from build123d import *

# Parameters (mm, degrees)
SKETCH1_W            = 93
SKETCH1_H            = 100
BOSS_EXTRUDE2_DEPTH  = 10
SKETCH4_W            = 10.01
SKETCH4_H            = 15
BOSS_EXTRUDE4_DEPTH  = 24
SKETCH5_R            = 2
CUT_EXTRUDE1_DEPTH   = 50
SKETCH7_R            = 11
CUT_EXTRUDE3_DEPTH   = 50
SKETCH14_W           = 61.5
SKETCH14_H           = 42
CUT_EXTRUDE8_DEPTH   = 4
SKETCH19_R           = 11
CUT_EXTRUDE11_DEPTH  = 15
SKETCH20_R           = 2
CUT_EXTRUDE12_DEPTH  = 10
SKETCH21_W           = 40
SKETCH21_H           = 6
BOSS_EXTRUDE5_DEPTH  = 27
SKETCH22_W           = 40
SKETCH22_H           = 6.3
BOSS_EXTRUDE7_DEPTH  = 40
SKETCH23_R           = 8
CUT_EXTRUDE13_DEPTH  = 40
SKETCH24_W           = 118.277817783
SKETCH24_H           = 41.8
CUT_EXTRUDE14_DEPTH  = 40
SKETCH25_W           = 31.5
SKETCH25_H           = 23.2
CUT_EXTRUDE15_DEPTH  = 20
CUT_EXTRUDE18_DEPTH  = 3
SKETCH27_R           = 4.1
SKETCH27_R_2         = 4
CUT_EXTRUDE29_DEPTH  = 3
SKETCH28_W           = 29.5
SKETCH28_H           = 58.2
CUT_EXTRUDE30_DEPTH  = 23
SKETCH29_W           = 32
SKETCH29_H           = 4
CUT_EXTRUDE31_DEPTH  = 23
SKETCH31_W           = 32
SKETCH31_H           = 6
BOSS_EXTRUDE9_DEPTH  = 6.6
SKETCH32_W           = 32
SKETCH32_H           = 6
BOSS_EXTRUDE10_DEPTH = 10
SKETCH33_R           = 2
CUT_EXTRUDE32_DEPTH  = 10
BOSS_EXTRUDE11_START = -32
BOSS_EXTRUDE11_DEPTH = 32
SKETCH35_R           = 3.5
CUT_EXTRUDE33_DEPTH  = 10
SKETCH36_W           = 27
SKETCH36_H           = 46
CUT_EXTRUDE34_DEPTH  = 50
SKETCH38_W           = 31.75
SKETCH38_H           = 35
CUT_EXTRUDE35_DEPTH  = 50
SKETCH40_W           = 4
SKETCH40_H           = 77.818306413
CUT_EXTRUDE37_DEPTH  = 110
SKETCH41_W           = 28
SKETCH41_H           = 1.72
CUT_EXTRUDE38_DEPTH  = 50
BOSS_EXTRUDE12_DEPTH = 30
SKETCH43_R           = 2
CUT_EXTRUDE39_DEPTH  = 30
SKETCH44_R           = 4.5
CUT_EXTRUDE40_DEPTH  = 3
SKETCH45_W           = 9.206702729
SKETCH45_H           = 6.861074725
SKETCH45_H_2         = 7.289433521
CUT_EXTRUDE41_DEPTH  = 3
SKETCH46_W           = 16
SKETCH46_H           = 27
CUT_EXTRUDE42_DEPTH  = 3
SKETCH47_R           = 2
CUT_EXTRUDE43_DEPTH  = 3
SKETCH48_R           = 3.5
CUT_EXTRUDE44_DEPTH  = 23


with BuildPart() as part:
    # Sketch1 → Boss-Extrude2 (new body)
    with BuildSketch(Plane.XY):
        with Locations((-29.68705036, 14.928057554)):
            Rectangle(SKETCH1_W, SKETCH1_H)
    extrude(amount=BOSS_EXTRUDE2_DEPTH)

    # Sketch4 → Boss-Extrude4 (add)
    with BuildSketch(Plane(origin=(16.81294964, 0, 0), x_dir=(0, 0, -1), z_dir=(1, 0, 0))):
        with Locations((-4.995, -12.571942446)):
            Rectangle(SKETCH4_W, SKETCH4_H)
    extrude(amount=BOSS_EXTRUDE4_DEPTH)

    # Sketch5 → Cut-Extrude1 (cut)
    with BuildSketch(Plane(origin=(0, -5.071942446, 0), x_dir=(1, 0, 0), z_dir=(0, 1, 0))):
        with Locations(Location((26.81294964, -5, 0), (0, 0, 180))):
            Circle(SKETCH5_R)
    extrude(amount=-CUT_EXTRUDE1_DEPTH, mode=Mode.SUBTRACT)

    # Sketch7 → Cut-Extrude3 (cut)
    with BuildSketch(Plane(origin=(0, 0, 0), x_dir=(-1, 0, 0), z_dir=(0, 0, -1))):
        with Locations((24.18705036, 36.928057554)):
            Circle(SKETCH7_R)
    extrude(amount=-CUT_EXTRUDE3_DEPTH, mode=Mode.SUBTRACT)

    # Sketch14 → Cut-Extrude8 (cut)
    with BuildSketch(Plane.XY.offset(10)):
        with Locations((-13.93705036, 36.789132279)):
            Rectangle(SKETCH14_W, SKETCH14_H)
    extrude(amount=-CUT_EXTRUDE8_DEPTH, mode=Mode.SUBTRACT)

    # Sketch19 → Cut-Extrude11 (cut)
    with BuildSketch(Plane(origin=(0, 0, 0), x_dir=(-1, 0, 0), z_dir=(0, 0, -1))):
        with Locations((53.18705036, 36.928057554)):
            Circle(SKETCH19_R)
    extrude(amount=-CUT_EXTRUDE11_DEPTH, mode=Mode.SUBTRACT)

    # Sketch20 → Cut-Extrude12 (cut)
    with BuildSketch(Plane.XY.offset(6)):
        with Locations((-34.68705036, 50.928057554)):
            Circle(SKETCH20_R)
        with Locations((5.31294964, 50.928057554)):
            Circle(SKETCH20_R)
        with Locations((-34.68705036, 22.928057554)):
            Circle(SKETCH20_R)
        with Locations((5.31294964, 22.928057554)):
            Circle(SKETCH20_R)
    extrude(amount=-CUT_EXTRUDE12_DEPTH, mode=Mode.SUBTRACT)

    # Sketch21 → Boss-Extrude5 (add)
    with BuildSketch(Plane(origin=(0, 0, 0), x_dir=(-1, 0, 0), z_dir=(0, 0, -1))):
        with Locations((56.18705036, 61.928057554)):
            Rectangle(SKETCH21_W, SKETCH21_H)
    extrude(amount=BOSS_EXTRUDE5_DEPTH)

    # Sketch22 → Boss-Extrude7 (add)
    with BuildSketch(Plane.XZ.offset(-58.928057554)):
        with Locations((-56.18705036, -23.85)):
            Rectangle(SKETCH22_W, SKETCH22_H)
    extrude(amount=BOSS_EXTRUDE7_DEPTH)

    # Sketch23 → Cut-Extrude13 (cut)
    with BuildSketch(Plane.XY.offset(10)):
        with Locations((-53.18705036, 36.928057554)):
            Circle(SKETCH23_R)
    extrude(amount=-CUT_EXTRUDE13_DEPTH, mode=Mode.SUBTRACT)

    # Sketch24 → Cut-Extrude14 (cut)
    with BuildSketch(Plane.XY.offset(10)):
        with Locations((-17.048141468, -14.171942446)):
            Rectangle(SKETCH24_W, SKETCH24_H)
    extrude(amount=-CUT_EXTRUDE14_DEPTH, mode=Mode.SUBTRACT)

    # Sketch25 → Cut-Extrude15 (cut)
    with BuildSketch(Plane.XY.offset(10)):
        with Locations((-60.43705036, 18.328057554)):
            Rectangle(SKETCH25_W, SKETCH25_H)
    extrude(amount=-CUT_EXTRUDE15_DEPTH, mode=Mode.SUBTRACT)

    # Sketch26 → Cut-Extrude18 (cut)
    with BuildSketch(Plane.XY.offset(6)):
        with BuildLine():
            Line((14.30212304, 57.789132279), (6.863398886, 57.789132279))
            Line((6.863398886, 57.789132279), (6.863398886, 54.615347499))
            ThreePointArc((6.863398886, 54.615347499), (8.24773413, 53.645968516), (9.108195728, 52.191428892))
            Line((9.108195728, 52.191428892), (14.30212304, 52.191428892))
            Line((14.30212304, 52.191428892), (14.30212304, 57.789132279))
        make_face()
        with BuildLine():
            Line((6.863398886, 19.240767609), (6.863398886, 15.789132279))
            Line((6.863398886, 15.789132279), (14.30212304, 15.789132279))
            Line((14.30212304, 15.789132279), (14.30212304, 20.928057554))
            Line((14.30212304, 20.928057554), (8.777051255, 20.928057554))
            ThreePointArc((8.777051255, 20.928057554), (7.95835451, 19.927752057), (6.863398886, 19.240767609))
        make_face()
        with BuildLine():
            Line((-36.237499605, 57.789132279), (-44.68705036, 57.789132279))
            Line((-44.68705036, 57.789132279), (-44.68705036, 52.191428892))
            Line((-44.68705036, 52.191428892), (-38.482296447, 52.191428892))
            ThreePointArc((-38.482296447, 52.191428892), (-37.621834849, 53.645968516), (-36.237499605, 54.615347499))
            Line((-36.237499605, 54.615347499), (-36.237499605, 57.789132279))
        make_face()
        with BuildLine():
            Line((-44.68705036, 21.664686216), (-44.68705036, 15.789132279))
            Line((-44.68705036, 15.789132279), (-36.237499605, 15.789132279))
            Line((-36.237499605, 15.789132279), (-36.237499605, 19.240767609))
            ThreePointArc((-36.237499605, 19.240767609), (-37.621834849, 20.210146592), (-38.482296447, 21.664686216))
            Line((-38.482296447, 21.664686216), (-44.68705036, 21.664686216))
        make_face()
    extrude(amount=-CUT_EXTRUDE18_DEPTH, mode=Mode.SUBTRACT)

    # Sketch27 → Cut-Extrude29 (cut)
    with BuildSketch(Plane.XY.offset(6)):
        with Locations((5.31294964, 50.928057554)):
            Circle(SKETCH27_R)
        with Locations((5.31294964, 22.928057554)):
            Circle(SKETCH27_R_2)
        with Locations((-34.68705036, 50.928057554)):
            Circle(SKETCH27_R)
        with Locations((-34.68705036, 22.928057554)):
            Circle(SKETCH27_R)
    extrude(amount=-CUT_EXTRUDE29_DEPTH, mode=Mode.SUBTRACT)

    # Sketch28 → Cut-Extrude30 (cut)
    with BuildSketch(Plane(origin=(0, 0, 0), x_dir=(-1, 0, 0), z_dir=(0, 0, -1))):
        with Locations((-2.06294964, 35.828057554)):
            Rectangle(SKETCH28_W, SKETCH28_H)
    extrude(amount=-CUT_EXTRUDE30_DEPTH, mode=Mode.SUBTRACT)

    # Sketch29 → Cut-Extrude31 (cut)
    with BuildSketch(Plane(origin=(0, 15.789132279, 0), x_dir=(1, 0, 0), z_dir=(0, 1, 0))):
        with Locations((-28.68705036, -8)):
            Rectangle(SKETCH29_W, SKETCH29_H)
    extrude(amount=-CUT_EXTRUDE31_DEPTH, mode=Mode.SUBTRACT)

    # Sketch31 → Boss-Extrude9 (add)
    with BuildSketch(Plane.XZ.offset(-6.728057554)):
        with Locations((-28.68705036, 3)):
            Rectangle(SKETCH31_W, SKETCH31_H)
    extrude(amount=BOSS_EXTRUDE9_DEPTH)

    # Sketch32 → Boss-Extrude10 (add)
    with BuildSketch(Plane.XY.offset(6)):
        with Locations((-28.68705036, 3.128057554)):
            Rectangle(SKETCH32_W, SKETCH32_H)
    extrude(amount=BOSS_EXTRUDE10_DEPTH)

    # Sketch33 → Cut-Extrude32 (cut)
    with BuildSketch(Plane(origin=(0, 6.128057554, 0), x_dir=(1, 0, 0), z_dir=(0, 1, 0))):
        with Locations(Location((-33.68705036, -11, 0), (0, 0, 270))):
            Circle(SKETCH33_R)
        with Locations(Location((-19.68705036, -11, 0), (0, 0, 270))):
            Circle(SKETCH33_R)
    extrude(amount=-CUT_EXTRUDE32_DEPTH, mode=Mode.SUBTRACT)

    # Sketch34 → Boss-Extrude11 (add)
    with BuildSketch(Plane(origin=(-12.68705036, 0, 0), x_dir=(0, 0, -1), z_dir=(1, 0, 0)).offset(BOSS_EXTRUDE11_START)):
        Polygon((-16, 6.128057554), (-6, 6.128057554), (-6, 14.058360342), align=None)
    extrude(amount=BOSS_EXTRUDE11_DEPTH)

    # Sketch35 → Cut-Extrude33 (cut)
    with BuildSketch(Plane.XZ.offset(-6.128057554)):
        with Locations((-19.68705036, 11)):
            Circle(SKETCH35_R)
        with Locations((-33.68705036, 11)):
            Circle(SKETCH35_R)
    extrude(amount=-CUT_EXTRUDE33_DEPTH, mode=Mode.SUBTRACT)

    # Sketch36 → Cut-Extrude34 (cut)
    with BuildSketch(Plane(origin=(-36.18705036, 0, 0), x_dir=(0, 0, -1), z_dir=(1, 0, 0))):
        with Locations((13.5, 41.928057554)):
            Rectangle(SKETCH36_W, SKETCH36_H)
    extrude(amount=-CUT_EXTRUDE34_DEPTH, mode=Mode.SUBTRACT)

    # Sketch38 → Cut-Extrude35 (cut)
    with BuildSketch(Plane.XY.offset(10)):
        with Locations((-60.31205036, 47.428057554)):
            Rectangle(SKETCH38_W, SKETCH38_H)
    extrude(amount=-CUT_EXTRUDE35_DEPTH, mode=Mode.SUBTRACT)

    # Sketch40 → Cut-Extrude37 (cut)
    with BuildSketch(Plane.XY.offset(16)):
        with Locations((-42.68705036, 39.037210761)):
            Rectangle(SKETCH40_W, SKETCH40_H)
    extrude(amount=-CUT_EXTRUDE37_DEPTH, mode=Mode.SUBTRACT)

    # Sketch41 → Cut-Extrude38 (cut)
    with BuildSketch(Plane.XY.offset(16)):
        with Locations((-26.68705036, 0.988057554)):
            Rectangle(SKETCH41_W, SKETCH41_H)
    extrude(amount=-CUT_EXTRUDE38_DEPTH, mode=Mode.SUBTRACT)

    # Sketch42 → Boss-Extrude12 (add)
    with BuildSketch(Plane(origin=(-12.68705036, 0, 0), x_dir=(0, 0, -1), z_dir=(1, 0, 0))):
        Polygon((-10, 64.928057554), (0, 64.928057554), (0, 1.848057554), (-16, 1.848057554), (-16, 6.128057554), (-6, 14.058360342), (-6, 57.789132279), (-10, 57.789132279), align=None)
    extrude(amount=BOSS_EXTRUDE12_DEPTH)

    # Sketch43 → Cut-Extrude39 (cut)
    with BuildSketch(Plane.XY.offset(6)):
        with Locations((5.31294964, 50.928057554)):
            Circle(SKETCH43_R)
        with Locations((5.31294964, 22.928057554)):
            Circle(SKETCH43_R)
    extrude(amount=-CUT_EXTRUDE39_DEPTH, mode=Mode.SUBTRACT)

    # Sketch44 → Cut-Extrude40 (cut)
    with BuildSketch(Plane.XY.offset(6)):
        with Locations((5.31294964, 22.928057554)):
            Circle(SKETCH44_R)
        with Locations((5.31294964, 50.928057554)):
            Circle(SKETCH44_R)
    extrude(amount=-CUT_EXTRUDE40_DEPTH, mode=Mode.SUBTRACT)

    # Sketch45 → Cut-Extrude41 (cut)
    with BuildSketch(Plane.XY.offset(6)):
        with Locations((12.709598275, 54.358594917)):
            Rectangle(SKETCH45_W, SKETCH45_H)
        with Locations((12.709598275, 18.736953601)):
            Rectangle(SKETCH45_W, SKETCH45_H_2)
    extrude(amount=-CUT_EXTRUDE41_DEPTH, mode=Mode.SUBTRACT)

    # Sketch46 → Cut-Extrude42 (cut)
    with BuildSketch(Plane.XY.offset(6)):
        with Locations((-4.607936524, 38.706325488)):
            Rectangle(SKETCH46_W, SKETCH46_H)
    extrude(amount=-CUT_EXTRUDE42_DEPTH, mode=Mode.SUBTRACT)

    # Sketch47 → Cut-Extrude43 (cut)
    with BuildSketch(Plane.XZ.offset(-1.848057554)):
        with Locations(Location((7.31294964, 11, 0), (0, 0, 270))):
            Circle(SKETCH47_R)
    extrude(amount=-CUT_EXTRUDE43_DEPTH, mode=Mode.SUBTRACT)

    # Sketch48 → Cut-Extrude44 (cut)
    with BuildSketch(Plane.XZ.offset(-4.848057554)):
        with Locations(Location((7.31294964, 11, 0), (0, 0, 270))):
            Circle(SKETCH48_R)
    extrude(amount=-CUT_EXTRUDE44_DEPTH, mode=Mode.SUBTRACT)


solid = part.part
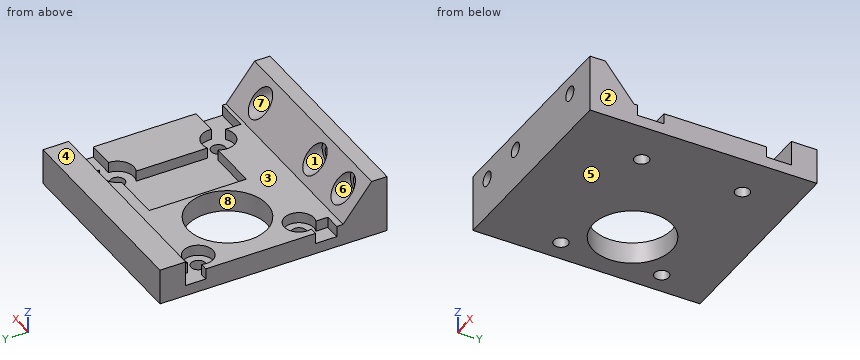
Input: part model. Units: mm. Frame: model coordinates. Face numbers are marked on the shaded views. A direction names the side the tool comes from. Round coordinates to 2 decimals unless told otherwise and drop trailing zeros. Order: outer loops, then holes, each group sorted by start corner. A loop starts at its lowest first (then second) coordinate and runs counter-clockwise, first axis right, second up.
1. Pin query (flat end, axial travel): P1, Ø8, axis at x = -35.5, y = 52.5, coming from the +Z side; P2, Ø6.5, axis at x = 5.31, y = 50.93, coming from the +Z side; P3, Ø2.5, axis at y = 55.5, z = 4.5, coming from the +X side. Return the tip coordinate at first contact, or that it passes through.
The answers:
P1: stops at z = 6
P2: stops at z = 3
P3: stops at x = 8.11
2. Set-up query: the marked faces 1, 2, 3 and 4. Return all of +Z, -Z, +X, -X, +Y, -Y with unobstructed straight access to the full face (end or side cutting, diameter ignored); none if empty.
The answers:
face 1: none
face 2: +Z, -Z, +X, +Y, -Y
face 3: +Z, +X, -X
face 4: +Z, +X, -X, +Y
3. Cut plane D-D, the plane y = 59. Output: boundary loops of the cut face in (x, z), then the cut area to 3 significant figures.
The answers:
outline: (-40.69, 0) - (17.31, 0) - (17.31, 10) - (-40.69, 10) - close
area: 580 mm2
4. Mould query, pull axis Z, two halves, no side actions, for the marked faces 5, 6, 7 and 8. Classes: released by +Z, released by -Z, zero draft, split by the parting line, or undercut.
The answers:
face 5: released by -Z
face 6: undercut
face 7: undercut
face 8: zero draft
5. Material intervals for line 1 (X direction, y = 2.6, z = 11); line 2 (X direction, y = 8.75, z = 11); line 3 (X direction, y = 35.5, z = 5.5), sorted ascending.
The answers:
line 1: x = -40.69 to -35.69, -31.69 to -21.69, -17.69 to 5.31, 9.31 to 17.31
line 2: x = -40.69 to -37.19, -30.19 to -23.19, -16.19 to 3.81, 10.81 to 17.31
line 3: x = -40.69 to -35.09, -13.28 to -12.61, 3.39 to 17.31
6. Cut plane C-C, the plane y = 9. Output: boundary loops of the cut face in (x, z), then the cut area to 3 significant figures.
The answers:
outline: (-40.69, 0) - (17.31, 0) - (17.31, 12.38) - (10.53, 12.38) arc R3.5 cw (long way) to (4.1, 12.38) - (-16.47, 12.38) arc R3.5 cw (long way) to (-22.9, 12.38) - (-30.47, 12.38) arc R3.5 cw (long way) to (-36.9, 12.38) - (-40.69, 12.38) - close
area: 632 mm2
7. Cut plane B-B, the plane z = 11. Output: boundary loops of the cut face in (x, y).
The answers:
outline: (-40.69, 1.85) - (-35.69, 1.85) - (-35.69, 6.13) - (-37.19, 6.13) - (-37.19, 10.09) - (-40.69, 10.09) - close; (-31.69, 1.85) - (-21.69, 1.85) - (-21.69, 6.13) - (-23.19, 6.13) - (-23.19, 10.09) - (-30.19, 10.09) - (-30.19, 6.13) - (-31.69, 6.13) - close; (-17.69, 1.85) - (5.31, 1.85) - (5.31, 4.85) - (3.81, 4.85) - (3.81, 10.09) - (-16.19, 10.09) - (-16.19, 6.13) - (-17.69, 6.13) - close; (9.31, 1.85) - (17.31, 1.85) - (17.31, 10.09) - (10.81, 10.09) - (10.81, 4.85) - (9.31, 4.85) - close
8. Cut plane A-A, the plane z = 4.25. State how many separate pieces and enclosed holes the cut face has, then the cut area to 3 significant figures.
The answers:
separate pieces: 2
enclosed holes: 1
area: 2,460 mm2
